```python
from build123d import *

# Parameters (mm, degrees)
SKETCH1_W                 = 73
SKETCH1_H                 = 7.715
BOSS_EXTRUDE1_DEPTH       = 6
SKETCH2_R                 = 0.5
BOSS_EXTRUDE2_DEPTH       = 1
SKETCH3_W                 = 0.35
SKETCH3_H                 = 2.54
BOSS_EXTRUDE3_DEPTH       = 2.5
SKETCH4_W                 = 0.325
SKETCH4_H                 = 2.5
BOSS_EXTRUDE4_DEPTH       = 2.54
BOSS_EXTRUDE12_DEPTH      = 5.715
BOSS_EXTRUDE12_DEPTH_BACK = 2
SKETCH13_W                = 12
SKETCH13_H                = 3.715
CUT_EXTRUDE1_DEPTH        = 39.025139382


with BuildPart() as part:
    # Sketch1 → Boss-Extrude1 (new body)
    with BuildSketch(Plane(origin=(0, 0, 0), x_dir=(1, 0, 0), z_dir=(0, 1, 0))):
        with Locations((0, -1.8575)):
            Rectangle(SKETCH1_W, SKETCH1_H)
    extrude(amount=BOSS_EXTRUDE1_DEPTH)

    # Sketch2 → Boss-Extrude2 (add)
    with BuildSketch(Plane(origin=(0, 6, 0), x_dir=(1, 0, 0), z_dir=(0, 1, 0))):
        with Locations(Location((2.25, 0, 0), (0, 0, 90))):
            Circle(SKETCH2_R)
        with Locations(Location((6.75, 0, 0), (0, 0, 90))):
            Circle(SKETCH2_R)
        with Locations(Location((11.25, 0, 0), (0, 0, 90))):
            Circle(SKETCH2_R)
        with Locations(Location((15.75, 0, 0), (0, 0, 90))):
            Circle(SKETCH2_R)
        with Locations(Location((20.25, 0, 0), (0, 0, 90))):
            Circle(SKETCH2_R)
        with Locations(Location((24.75, 0, 0), (0, 0, 90))):
            Circle(SKETCH2_R)
        with Locations(Location((29.25, 0, 0), (0, 0, 90))):
            Circle(SKETCH2_R)
        with Locations(Location((33.75, 0, 0), (0, 0, 90))):
            Circle(SKETCH2_R)
        with Locations(Location((-33.75, 0, 0), (0, 0, 90))):
            Circle(SKETCH2_R)
        with Locations(Location((-29.25, 0, 0), (0, 0, 90))):
            Circle(SKETCH2_R)
        with Locations(Location((-24.75, 0, 0), (0, 0, 90))):
            Circle(SKETCH2_R)
        with Locations(Location((-20.25, 0, 0), (0, 0, 90))):
            Circle(SKETCH2_R)
        with Locations(Location((-15.75, 0, 0), (0, 0, 90))):
            Circle(SKETCH2_R)
        with Locations(Location((-11.25, 0, 0), (0, 0, 90))):
            Circle(SKETCH2_R)
        with Locations(Location((-6.75, 0, 0), (0, 0, 90))):
            Circle(SKETCH2_R)
        with Locations(Location((-2.25, 0, 0), (0, 0, 90))):
            Circle(SKETCH2_R)
    extrude(amount=BOSS_EXTRUDE2_DEPTH)

    # Sketch3 → Boss-Extrude3 (add)
    with BuildSketch(Plane(origin=(0, 6, 0), x_dir=(1, 0, 0), z_dir=(0, 1, 0))):
        with Locations((4.5, -4.445)):
            Rectangle(SKETCH3_W, SKETCH3_H)
        with Locations((0, -4.445)):
            Rectangle(SKETCH3_W, SKETCH3_H)
        with Locations((9, -4.445)):
            Rectangle(SKETCH3_W, SKETCH3_H)
        with Locations((13.5, -4.445)):
            Rectangle(SKETCH3_W, SKETCH3_H)
        with Locations((18, -4.445)):
            Rectangle(SKETCH3_W, SKETCH3_H)
        with Locations((22.5, -4.445)):
            Rectangle(SKETCH3_W, SKETCH3_H)
        with Locations((27, -4.445)):
            Rectangle(SKETCH3_W, SKETCH3_H)
        with Locations((31.5, -4.445)):
            Rectangle(SKETCH3_W, SKETCH3_H)
        with Locations((36, -4.445)):
            Rectangle(SKETCH3_W, SKETCH3_H)
        with Locations((-4.5, -4.445)):
            Rectangle(SKETCH3_W, SKETCH3_H)
        with Locations((-9, -4.445)):
            Rectangle(SKETCH3_W, SKETCH3_H)
        with Locations((-13.5, -4.445)):
            Rectangle(SKETCH3_W, SKETCH3_H)
        with Locations((-18, -4.445)):
            Rectangle(SKETCH3_W, SKETCH3_H)
        with Locations((-22.5, -4.445)):
            Rectangle(SKETCH3_W, SKETCH3_H)
        with Locations((-27, -4.445)):
            Rectangle(SKETCH3_W, SKETCH3_H)
        with Locations((-31.5, -4.445)):
            Rectangle(SKETCH3_W, SKETCH3_H)
        with Locations((-36, -4.445)):
            Rectangle(SKETCH3_W, SKETCH3_H)
    extrude(amount=BOSS_EXTRUDE3_DEPTH)

    # Sketch4 → Boss-Extrude4 (add)
    with BuildSketch(Plane.XY.offset(3.175)):
        with Locations((-36.3375, 7.25)):
            Rectangle(SKETCH4_W, SKETCH4_H)
        with Locations((36.3375, 7.25)):
            Rectangle(SKETCH4_W, SKETCH4_H)
    extrude(amount=BOSS_EXTRUDE4_DEPTH)

    # Sketch12 → Boss-Extrude12 (add, two sides: drawn at the far end of the back side and taken through both)
    with BuildSketch(Plane.XY.offset(-BOSS_EXTRUDE12_DEPTH_BACK)):
        with BuildLine():
            Line((-2.54, -6), (-2.54, -9))
            Line((-2.54, -9), (-6, -9))
            Line((-6, -9), (-6, 0))
            Line((-6, 0), (6, 0))
            Line((6, 0), (6, -9))
            Line((6, -9), (2.54, -9))
            Line((2.54, -9), (2.54, -6))
            ThreePointArc((2.54, -6), (0, -3.46), (-2.54, -6))
        make_face()
    extrude(amount=BOSS_EXTRUDE12_DEPTH + BOSS_EXTRUDE12_DEPTH_BACK)

    # Sketch13 → Cut-Extrude1 (cut, through all)
    with BuildSketch(Plane.XZ):
        with Locations((0, 1.8575)):
            Rectangle(SKETCH13_W, SKETCH13_H)
    extrude(amount=CUT_EXTRUDE1_DEPTH, mode=Mode.SUBTRACT)


solid = part.part
```
Build history of the part. All positions in model axes, mm. A direction names the side the tool comes from. Round coordinates to 2 decimals unless told otherwise and drop trailing zeros. Loops run counter-clockwise (first coordinate to the right, second up) from the corner with the lowest first, then second, coordinate; pieces in that order, holes last. Notation, with made-up numbers: M 45.5,10 L 93.5,10 A7 ccw 93.5,15 Z; hole C 27,68.25 d10. An arc over 180 degrees is marked long. Answer as CSV lines item,"result".
1. Wall check: probe 1 along X at (y, z) = (-6.5, -0.75); probe 2 along Y at (x, z) = (17, 1.25); probe 3 along X at (y, z) = (-3.75, -0.75). Give the ranges that are in metal, low to high. Write a range as [from, to].
Resolved:
probe 1,"x = [-6, -2.54], [2.54, 6]"
probe 2,"y = [0, 6]"
probe 3,"x = [-6, -1.18], [1.18, 6]"
2. 3-axis set-ups, long thin cutter, end or side, ignore diameter. For faces 4 (the flat face through (2.54, -8, -1)), 5 (the flat face through (-4, -9, -1)), 6 (the flat face through (-8.825, 7, 4)): which of +Z, -Z, +X, -X, +Y, -Y reach the whole face in a straight line?
Resolved:
face 4,"+Z, -Z, -Y"
face 5,"+Z, -Z, +X, -X, -Y"
face 6,"+Z, -Z, +Y"
3. Flat gauge pins, fed straight in: P1, Ø0.8, axis at x = 2.5, z = 0, coming from the +Y side; P2, Ø1.5, axis at y = -2, z = 3, coming from the -X side. Where does each tip first touch, or does it go through?
Resolved:
P1,"stops at y = 7"
P2,"stops at x = -6"
4. Cut at B-B on z = 2. Write the cut outline in (x, y).
Resolved:
outline,"M -36.5,0 L 36.5,0 L 36.5,6 L -36.5,6 Z"
5. Cut at A-A on y = -2.75. Write the cut outline in (x, z) (3 decimals), then the cut area to 3 significant figures.
Resolved:
outline,"M -6,-2 L 6,-2 L 6,0 L -6,0 Z; M -6,3.715 L 6,3.715 L 6,5.715 L -6,5.715 Z"
area,"48.0 mm²"
6. Two-plate mould, pull along X, no slides. Class faces 1 (the flat face through (-4, -9, 5)), 2 (the flat face through (27.175, 7, 4)), 3 (the cylindrical face through (0.06, -3.46, 4.7)): released by +X, released by -X, zero draft, split by the parting line, or undercut.
Resolved:
face 1,"zero draft"
face 2,"undercut"
face 3,"undercut"
